Here's the drawing with two shaded views (mm, measured from the low corner). I have some questions. A direction names the side the tool comes from. Round coordinates to 2 decimals unless told otherwise and drop trailing zeros. Write each loop counter-clockwise with the first axis right and the second up, starting at its lowest first coordinate (ties: lowest second). Pieces come first, ordered by that corner, then holes. Notation, with made-up numbers: M -34,22 L -14,22 A10 cw -14,37 Z; hole C 53,-21 d4. An arc over 180 degrees is marked long. Answer as a JSON object with one key per item and string values. Group by question number.
1) On a 3-axis mill with a long thin cutter (end or side, diameter ignored), from which of +Z, -Z, +X, -X, +Y, -Y can I reach the whole of each face in a straight line? I mean the marked faces 4 and 5. Say none if no direction works.
2) Suppose I cut it at A-A, the plane y = 900. Write out the boundary of the cut face in (x, z).
3) Suppose I cut it at C-C, the plane z = 601. Write out the boundary of the cut face in (x, y), and give its area (3 significant figures).
4) Suppose I cut it at D-D, the plane x = 256. Write out the boundary of the cut face in (y, z), and give its area (3 significant figures).
5) Please list where these lines run through material, in increasing order: L1, parallel to Z at x = 672, y = 961; L2, parallel to X at y = 911, z = 362.5; L3, parallel to Z at x = 1377, y = 1285.5. Write a range as [from, to].
6) If we mould it in two halves opening along Z, with no side actions, what happens to the marked faces 1, 2 and 3? For each: +Z half, -Z half, draft (parallel to the pull), parting line (faces both ways), or undercut.
7) I'm going to push flat-ended pins straight in: pin 1 Ø2 at (x, y) = (1426.5, 236.5) entering from -Z; pin 2 Ø15 at (x, z) = (810.5, 29) entering from -Y; pin 3 Ø3 at (y, z) = (895, 154) entering from -X. Where does each tip first touch, or does it pass through?
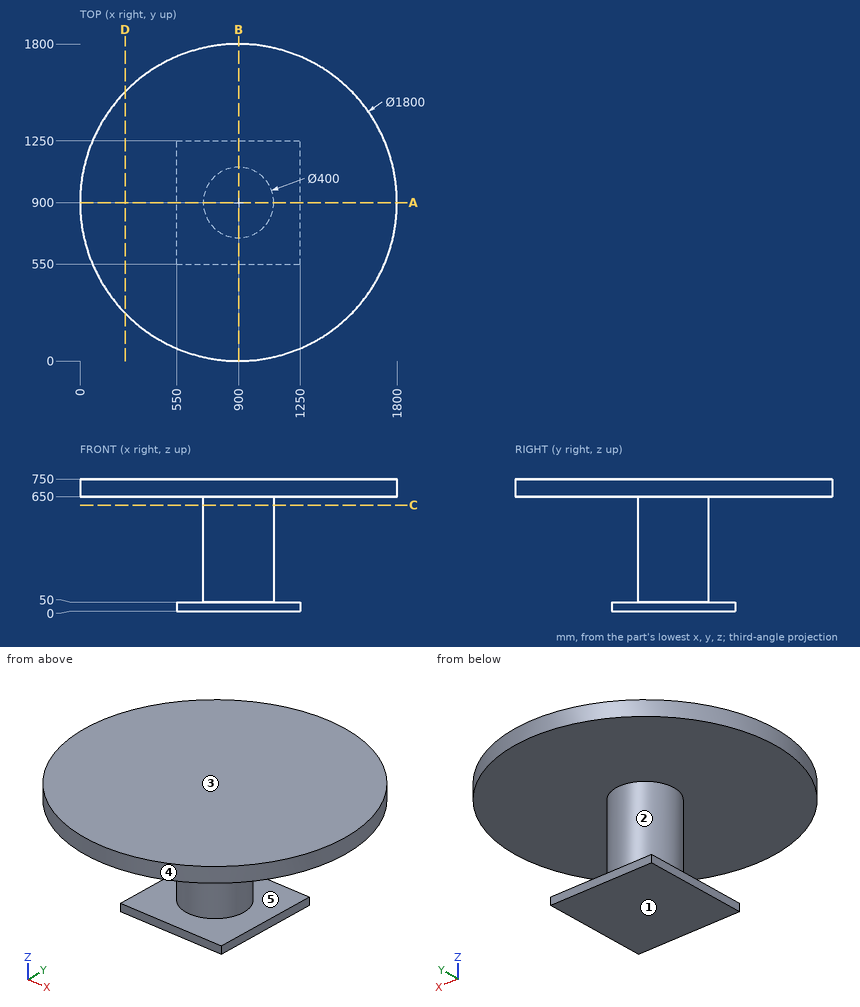
Results:
{
 "1": {"face 4": "+Z, -Z", "face 5": "none"},
 "2": {"outline": "M 0,650 L 700,650 L 700,50 L 550,50 L 550,0 L 1250,0 L 1250,50 L 1100,50 L 1100,650 L 1800,650 L 1800,750 L 0,750 Z"},
 "3": {"outline": "C 900,900 d400", "area": "126,000 mm^2"},
 "4": {"outline": "M 271.3,650 L 1528.7,650 L 1528.7,750 L 271.3,750 Z", "area": "126,000 mm^2"},
 "5": {"L1": "[0, 50], [650, 750]", "L2": "[700.3, 1099.7]", "L3": "[650, 750]"},
 "6": {"face 1": "-Z half", "face 2": "undercut", "face 3": "+Z half"},
 "7": {"pin 1": "z = 650", "pin 2": "y = 550", "pin 3": "x = 700.03"}
}
